```python
from build123d import *

# Parameters (mm, degrees)
F0_W     = 120
F0_H     = 80
F1_DEPTH = 4
F2_W     = 69
F2_H     = 68.5
F3_DEPTH = 5
F4_SIZE2 = 4.99999
F4_SIZE  = 1.49999


# Not quite as in the source:
# - a fillet or chamfer is up to 0.001 mm smaller than in the source, because OpenCascade refuses the exact size


with BuildPart() as f1:
    # F0 (on Top) → F1 (new body)
    with BuildSketch(Plane.XY):
        Rectangle(F0_W, F0_H)
    extrude(amount=F1_DEPTH)

    # F2 (on face) → F3 (join)
    with BuildSketch(Plane.XY.offset(4)):
        Rectangle(F2_W, F2_H)
    extrude(amount=F3_DEPTH)

    # F4 (size 1.5 and 5 in the source; OpenCascade refuses exactly that, so slightly less here)
    f4_edges = [f1.edges().sort_by_distance(p)[0] for p in [
        (0, 34.25, 9),
        (0, -34.25, 9),
    ]]
    f4_side = f1.faces().sort_by_distance((0, 0, 9))[0]
    chamfer(f4_edges, length=F4_SIZE, length2=F4_SIZE2, reference=f4_side)


solid = f1.part
```
The model under review builds one solid part; all positions refer to its coordinate system, in mm. A direction names the side the tool comes from. Give positions to 0.01 mm unless a question says otherwise; leave off trailing zeros. Write each loop counter-clockwise with the first axis right and the second up, starting at its lowest first coordinate (ties: lowest second). Pieces come first, ordered by that corner, then holes. Notation, with made-up numbers: M 66,-24 L 82,-24 A27 cw 82,-1 Z; hole C 66,6 d11. An arc over 180 degrees is marked long. Answer in a Markdown table with one row per item.
Item 1: Add section D-D on x = 45. Give the boundary of the cut face in (y, z).
Check sheet entries:
| item | result |
|---|---|
| outline | M -40,0 L 40,0 L 40,4 L -40,4 Z |
Item 2: Tool access review of faces 1 (the face through (34.5, 0, 6)), 2 (the face through (-34.5, 0, 6)), 3 (the face through (-60, -1, 2)): name each direction out of +Z, -Z, +X, -X, +Y, -Y from which nothing blocks a thin tool from reaching the whole face with its end or side.
Check sheet entries:
| item | result |
|---|---|
| face 1 | +Z, +X, +Y, -Y |
| face 2 | +Z, -X, +Y, -Y |
| face 3 | +Z, -Z, -X, +Y, -Y |
Item 3: For line 1 along X through (y, z) = (0, 4.25); line 2 along Z through (x, y) = (-46, -35.5); line 3 along Y through (x, z) = (-4, 4.25) (3 decimals), list the stretches that pass through material, from the lowest coordinate up.
Check sheet entries:
| item | result |
|---|---|
| line 1 | -34.5 to 34.5 |
| line 2 | 0 to 4 |
| line 3 | -34.175 to 34.175 |
Item 4: For P1, Ø1.5, axis at y = 3, z = 7, coming from the +X side; P2, Ø1.5, axis at y = 31.5, z = 8, coming from the -X side, all flat-tipped, find the tip position at first contact; note any pin that passes through.
Check sheet entries:
| item | result |
|---|---|
| P1 | x = 34.5 |
| P2 | x = -34.5 |
Item 5: Add section B-B on y = -26.5. Give the boundary of the cut face in (x, z), plus the area to 3 significant figures.
Check sheet entries:
| item | result |
|---|---|
| outline | M -60,0 L 60,0 L 60,4 L 34.5,4 L 34.5,9 L -34.5,9 L -34.5,4 L -60,4 Z |
| area | 825 mm2 |
Item 6: Add section C-C on z = 6. Give the boundary of the cut face in (x, y), plus the area to 3 significant figures.
Check sheet entries:
| item | result |
|---|---|
| outline | M -34.5,-33.65 L 34.5,-33.65 L 34.5,33.65 L -34.5,33.65 Z |
| area | 4,640 mm2 |
